Input: part model. Units: mm. Frame: model coordinates. A direction names the side the tool comes from. Round coordinates to 2 decimals unless told otherwise and drop trailing zeros. Write each loop counter-clockwise with the first axis right and the second up, starting at its lowest first coordinate (ties: lowest second). Pieces come first, ordered by that corner, then holes. Notation, with made-up numbers: (70, -6) - (92, -6) arc R20 ccw to (92, 1) - close; hole circle Ø8 at (-28, 51.25). An arc over 180 degrees is marked (long way). Use one line per item in the form item = value.
```python
from build123d import *

# Parameters (mm, degrees)
F1_DEPTH = 56.515
F3_D     = 7.366
F3_DEPTH = 10.16
F4_D     = 7.366
F4_DEPTH = 10.16


with BuildPart() as f1:
    # F0 (on Front) → F1 (new body)
    with BuildSketch(Plane.XZ):
        Polygon((27.94, 0), (10.16, 0), (10.16, 10.16), (0, 10.16), (0, 0), (0, -12.7), (85.09, -12.7), (85.09, 0), (85.09, 24.900328), (78.959122, 24.900328), (78.959122, 0), (40.64, 0), (40.64, 33.02), (27.94, 33.02), align=None)
    extrude(amount=F1_DEPTH)

    # F3
    with Locations(Plane.YZ.offset(85.09)):
        with Locations((-37.39713, 13.904383)):
            Hole(F3_D / 2, depth=F3_DEPTH)

    # F4
    with Locations(Plane.YZ.offset(85.09)):
        with Locations((-14.272088, 13.904383)):
            Hole(F4_D / 2, depth=F4_DEPTH)


solid = f1.part
```
(1) Cut plane D-D on z = 27. Output: boundary loops of the cut face in (x, y) (3 decimals), then the cut area to 3 significant figures.
Derived:
outline = (27.94, -56.515) - (40.64, -56.515) - (40.64, 0) - (27.94, 0) - close
area = 718 mm^2
(2) Cut plane A-A on z = 3.5. Output: boundary loops of the cut face in (x, y) (3 decimals).
Derived:
outline = (0, -56.515) - (10.16, -56.515) - (10.16, 0) - (0, 0) - close; (27.94, -56.515) - (40.64, -56.515) - (40.64, 0) - (27.94, 0) - close; (78.959, -56.515) - (85.09, -56.515) - (85.09, 0) - (78.959, 0) - close
(3) Material intervals for L1, parallel to X at y = -6, z = 8.5; L2, parallel to X at y = -16, z = 21; L3, parallel to X at y = -23, z = 29, sorted ascending.
Derived:
L1 = 0 to 10.16, 27.94 to 40.64, 78.96 to 85.09
L2 = 27.94 to 40.64, 78.96 to 85.09
L3 = 27.94 to 40.64
(4) Draft query along Z for faces 6 (the face through (42, -56.515, -5)), 7 (the face through (81.98, -16.25, 17.01)), 8 (the face through (42, -28, -12.7)). Return one class per face: released by +Z, released by -Z, zero draft, split by the parting line, or undercut.
Derived:
face_6 = zero draft
face_7 = undercut
face_8 = released by -Z
(5) First-contact query: pin 1 Ø7.5 at (y, z) = (-32, 15) entering from -X; pin 2 Ø3 at (x, y) = (54, -34.5) entering from +Z; pin 3 Ø3 at (x, y) = (82.5, -28) entering from +Z. Flat tips, straight axial feed; report the tip coordinate or a pass-through.
Derived:
pin_1 = 27.94
pin_2 = 0
pin_3 = 24.9
(6) Cut plane C-C on y = -13.5. Output: boundary loops of the cut face in (x, z), then the cut area to 3 significant figures.
Derived:
outline = (0, -12.7) - (85.09, -12.7) - (85.09, 10.3) - (78.96, 10.3) - (78.96, 0) - (40.64, 0) - (40.64, 33.02) - (27.94, 33.02) - (27.94, 0) - (10.16, 0) - (10.16, 10.16) - (0, 10.16) - close; (78.96, 17.51) - (85.09, 17.51) - (85.09, 24.9) - (78.96, 24.9) - close
area = 1,710 mm^2
(7) Access query for faces 1 (the face through (5, -28, 10.16)), 2 (the face through (82, -28, 24.9)), 3 (the face through (81.98, -40.91, 15.01)), 4 (the face through (27.94, -28, 17)), 5 (the face through (42, 0, -5)). Directions: +Z, -Z, +X, -X, +Y, -Y. A direction counts if a zero-diameter tool reaches every point of the face in a straight line with its end or side. Return the directions, or none.
Derived:
face_1 = +Z, -X, +Y, -Y
face_2 = +Z, +X, +Y, -Y
face_3 = +X
face_4 = +Z, +Y, -Y
face_5 = +Z, -Z, +X, -X, +Y
(8) Cut plane B-B on y = -21. Output: boundary loops of the cut face in (x, z), then the cut area to 3 significant figures.
Derived:
outline = (0, -12.7) - (85.09, -12.7) - (85.09, 24.9) - (78.96, 24.9) - (78.96, 0) - (40.64, 0) - (40.64, 33.02) - (27.94, 33.02) - (27.94, 0) - (10.16, 0) - (10.16, 10.16) - (0, 10.16) - close
area = 1,760 mm^2
